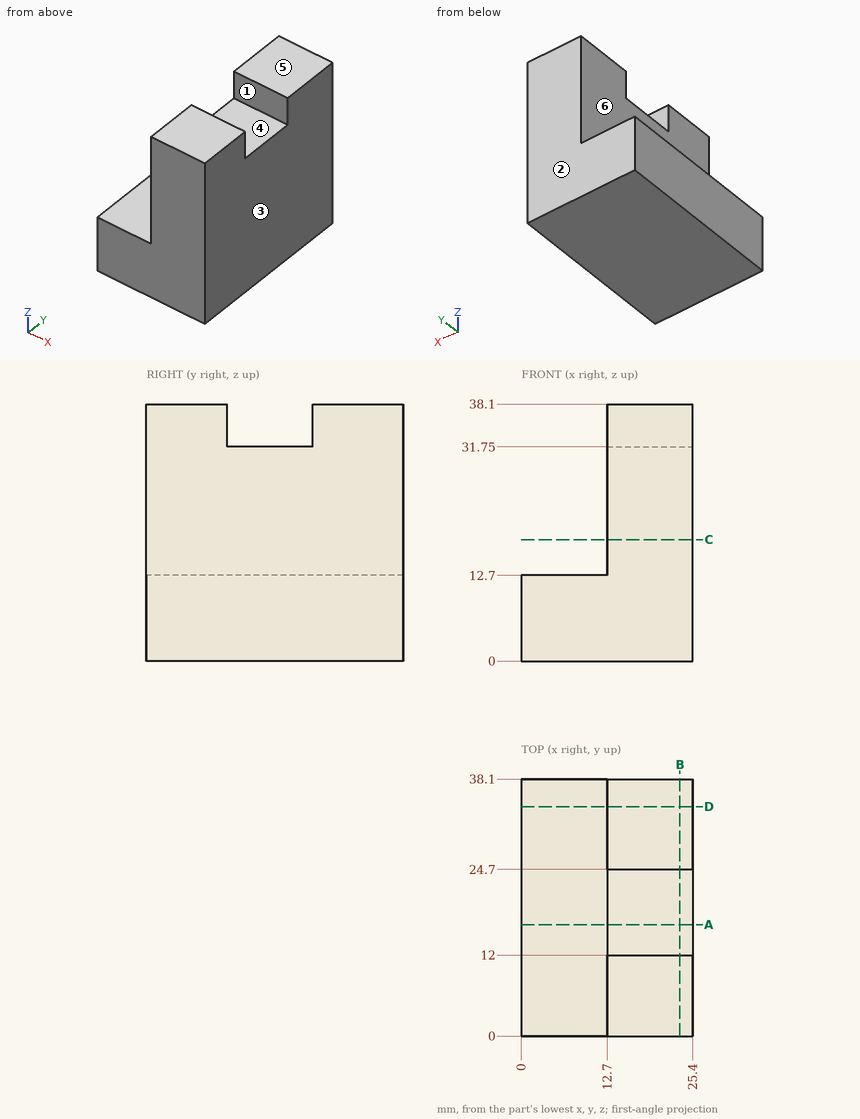
Check sheet for the drawn part. Datum: minimum x, y, z corner. Units: mm. A direction names the side the tool comes from. Give positions to 0.01 mm unless a question says otherwise; leave off trailing zeros. Order: outer loops, then holes, each group sorted by start corner. A loop starts at its lowest first (then second) coordinate and runs counter-clockwise, first axis right, second up. Notation, with made-up numbers: (46, 70.5) - (62, 70.5) arc R14 ccw to (62, 93.5) - close; hole circle Ø10 at (-32, 73). An arc over 180 degrees is marked (long way). Answer in a Markdown table with one row per item. Add a question column.
Q1. Cross-section at D-D, the plane y = 34. Enter the section's corners in (x, z), then the cut area to 3 significant figures.
Q2. Material ranges on probe 1 along Y at (x, z) = (18.5, 36.5); probe 2 along Z at (x, y) = (19.25, 19.5); probe 3 along X at (y, z) = (27.5, 34.5), recorded low to high. Write a range as from..to.
Q3. Mould release check, pull along Y, two halves, no side actions. Record for the marked faces 1, 2, 3 and 4: pulls with the +Y half, pulls with the -Y half, needs draft (parallel to the pull), parting line crosses it, or undercut.
Q4. Cross-section at B-B, the plane x = 23.5. Enter the section's corners in (y, z).
Q5. Tool access check on the marked faces 5 and 6. Record the directions out of +Z, -Z, +X, -X, +Y, -Y that give a thin tool (end or side, any length) a straight path to the whole face; none if there is none.
Q6. Cross-section at C-C, the plane z = 18. Enter the section's corners in (x, y).
Q7. Gauge pin test, flat ends, axial feed: pin 1 (2 mm diameter, centred on x = 17, y = 20.5, fed in from +Z); pin 2 (4 mm diameter, centred on x = 7, y = 24, fed in from +Z); pin 3 (7.5 mm diameter, centred on y = 19.5, z = 27, fed in from -X). Record the tip position at first contact, or that the pin passes through.
Q8. Cross-section at A-A, the plane y = 16.5. Enter the section's corners in (x, z).
Check values:
| question | item | result |
|---|---|---|
| 1 | outline | (0, 0) - (25.4, 0) - (25.4, 38.1) - (12.7, 38.1) - (12.7, 12.7) - (0, 12.7) - close |
| 1 | area | 645 mm^2 |
| 2 | probe 1 | y = 0..12, 24.7..38.1 |
| 2 | probe 2 | z = 0..31.75 |
| 2 | probe 3 | x = 12.7..25.4 |
| 3 | face 1 | undercut |
| 3 | face 2 | pulls with the +Y half |
| 3 | face 3 | needs draft |
| 3 | face 4 | undercut |
| 4 | outline | (0, 0) - (38.1, 0) - (38.1, 38.1) - (24.7, 38.1) - (24.7, 31.75) - (12, 31.75) - (12, 38.1) - (0, 38.1) - close |
| 5 | face 5 | +Z, +X, -X, +Y, -Y |
| 5 | face 6 | +Z, -X, +Y, -Y |
| 6 | outline | (12.7, 0) - (25.4, 0) - (25.4, 38.1) - (12.7, 38.1) - close |
| 7 | pin 1 | stops at z = 31.75 |
| 7 | pin 2 | stops at z = 12.7 |
| 7 | pin 3 | stops at x = 12.7 |
| 8 | outline | (0, 0) - (25.4, 0) - (25.4, 31.75) - (12.7, 31.75) - (12.7, 12.7) - (0, 12.7) - close |
